Autodesk Inventor part; units mm, degrees
ref_plane "YZ Plane" through (0, 0, 0) normal (1, 0, 0) x (0, 1, 0)
ref_plane "XZ Plane" through (0, 0, 0) normal (0, 1, 0) x (-1, 0, 0)
ref_plane "XY Plane" through (0, 0, 0) normal (0, 0, 1) x (1, 0, 0)
sketch "Sketch1" plane through (0, 0, 0) normal (0, 0, 1) x (1, 0, 0)
  line L0 (-24.6491, 25.3024) -> (-4.9641, 25.3024)
  line L1 (-4.9641, 25.3024) -> (-4.9641, -19.1476)
  line L2 (-4.9641, -19.1476) -> (-24.6491, -19.1476)
  line L3 (-24.6491, -19.1476) -> (-24.6491, 25.3024)
  point P0 (0, 0)
  dimension "d0" = 19.685
  dimension "d1" = 44.45
extrude "Extrusion1" add sketch "Sketch1" along normal blind 12.7
sketch "Sketch2" plane through (0, 0, 12.7) normal (0, 0, 1) x (1, 0, 0)
  line L0 (-4.9641, 25.3024) -> (-4.9641, -19.1476)
  line L1 (-24.6491, -19.1476) -> (-4.9641, -19.1476)
  line L2 (-4.9641, -19.1476) -> (-4.9641, 12.577)
  line L3 (-4.9641, 12.577) -> (-24.6491, 12.577)
  line L4 (-24.6491, 12.577) -> (-24.6491, -19.1476)
  point P0 (0, 0)
  dimension "d4" = 31.7246
extrude "Extrusion2" add sketch "Sketch2" along normal blind 9.7282
sketch "Sketch3" plane through (0, 0, 22.4282) normal (0, 0, 1) x (1, 0, 0)
  line L0 (-24.6491, 12.577) -> (-4.9641, 12.577)
  line L1 (-4.9641, 12.577) -> (-7.9613, 12.577)
  line L2 (-7.9613, 12.577) -> (-7.9613, 9.5798)
  line L3 (-24.6491, 12.577) -> (-21.6519, 12.577)
  line L4 (-21.6519, 12.577) -> (-21.6519, 9.5798)
  point P0 (0, 0)
  dimension "d7" = 2.9972
  dimension "d8" = 2.9972
  dimension "d9" = 2.9972
  dimension "d10" = 2.9972
hole "Hole1" at (-21.6519, 9.5798, 22.4282) at (-7.9613, 9.5798, 22.4282) direction (0, 0, -1) diameter 2.4892 depth 12.7 tip angle 118
sketch "Sketch4" plane through (0, 0, 12.7) normal (0, 0, 1) x (1, 0, 0)
  line L0 (-24.6491, 12.577) -> (-4.9641, 12.577)
  line L1 (-24.6491, 25.3024) -> (-4.9641, 25.3024)
  line L2 (-14.8066, 25.3024) -> (-14.8066, 12.577)
  line L3 (-14.8066, 18.9397) -> (-10.9966, 18.9397)
  line L4 (-14.8066, 18.9397) -> (-18.6166, 18.9397)
  point P0 (0, 0)
  dimension "d18" = 3.81
  dimension "d19" = 3.81
hole "Hole2" at (-10.9966, 18.9397, 12.7) at (-18.6166, 18.9397, 12.7) direction (0, 0, -1) diameter 3.81 depth 12.7 tip angle 118
properties part number "X+Z axis home sensor block"
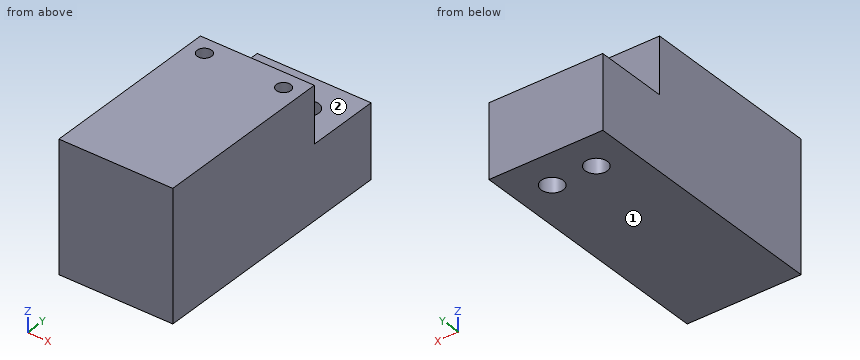
Work out the finished part from the listing and answer in its coordinate system (mm). Face numbers are marked on the shaded views. A direction names the side the tool comes from. Coordinates: 2 decimals unless noted, no trailing zeros. Write each loop counter-clockwise with the first axis right and the second up, starting at its lowest first coordinate (ties: lowest second). Pieces come first, ordered by that corner, then holes. Notation, with made-up numbers: (73.25, 12.25) - (123.25, 12.25) arc R11 ccw to (123.25, 16.25) - close; hole circle Ø2 at (69.25, 79.25). An arc over 180 degrees is marked (long way). Answer as a JSON object with one key per item and string values.
Q1. Which of the six approach directions +Z, -Z, +X, -X, +Y, -Y give full straight-line access (tool end or side, diameter ignored) to the marked faces 1 and 2?
Results list:
{"face 1": "-Z, +X, -X, +Y, -Y", "face 2": "+Z, +X, -X, +Y"}
Q2. Given pin 1 Ø3 at (x, z) = (-10, 19.5) entering from +Y; pin 2 Ø3.5 at (x, y) = (-11, 18.94) entering from +Z, each flat-ended and moving along its own axis, determine where each tip first touches the part or whether it passes through.
Results list:
{"pin 1": "stops at y = 12.58", "pin 2": "passes through"}
Q3. Find section D-D (y = 15.5). Write down the section's boundary in (x, z), plus the area to 3 significant figures.
Results list:
{"outline": "(-24.65, 0) - (-4.96, 0) - (-4.96, 12.7) - (-24.65, 12.7) - close", "area": "250 mm^2"}
Q4. Consider L1, parallel to Y at x = -18.5, z = 8.5; L2, parallel to Y at x = -18.5, z = 19.25; L3, parallel to Z at x = -16.75, y = 13. Determine where each line is inside the solid, lowest interval first. Write a range as from..to.
Results list:
{"L1": "y = -19.15..17.04, 20.84..25.3", "L2": "y = -19.15..12.58", "L3": "z = 0..12.7"}
Q5. Find section A-A (z = 12.25). Write down the section's boundary in (x, y) (3 decimals).
Results list:
{"outline": "(-24.649, -19.148) - (-4.964, -19.148) - (-4.964, 25.302) - (-24.649, 25.302) - close; hole circle Ø2.489 at (-21.652, 9.58); hole circle Ø3.81 at (-18.617, 18.94); hole circle Ø3.81 at (-10.997, 18.94); hole circle Ø2.489 at (-7.961, 9.58)"}
Q6. Find section B-B (x = -16). Write down the section's boundary in (y, z).
Results list:
{"outline": "(-19.15, 0) - (25.3, 0) - (25.3, 12.7) - (12.58, 12.7) - (12.58, 22.43) - (-19.15, 22.43) - close"}
Q7. Find section C-C (x = -18). Write down the section's boundary in (y, z).
Results list:
{"outline": "(-19.15, 0) - (17.14, 0) - (17.14, 12.7) - (12.58, 12.7) - (12.58, 22.43) - (-19.15, 22.43) - close; (20.74, 0) - (25.3, 0) - (25.3, 12.7) - (20.74, 12.7) - close"}
